from build123d import *

# Parameters (mm, degrees)
F0_W     = 25.4
F0_H     = 25.4
F1_DEPTH = 101.6
F3_DEPTH = 4.7625
F5_COUNT = 4
F5_ANGLE = 270


with BuildPart() as f1:
    # F0 (on Top) → F1 (new body)
    with BuildSketch(Plane.XY):
        Rectangle(F0_W, F0_H)
    extrude(amount=-F1_DEPTH)

    # F2 (on Right) → F3 (join, symmetric)
    with BuildSketch(Plane.YZ):
        Polygon((-88.9, -101.6), (-12.7, -101.6), (-12.7, -63.5), (-88.9, -95.25), align=None)
        Polygon((-15.3570100665, -67.4855150998), (-15.3570100665, -98.9429899335), (-86.2429899335, -98.9429899335), (-86.2429899335, -97.0213400443), align=None, mode=Mode.SUBTRACT)
    extrude(amount=F3_DEPTH, both=True)

    # F5: F1 ×4 about axis
    f5_axis = Axis((0, 0, -52.7451187372), (0, 0, -1))


with BuildPart() as f1_1:
    add(f1.part)
    for i in range(1, F5_COUNT):
        add(f1.part.rotate(f5_axis, i * F5_ANGLE / (F5_COUNT - 1)))


solid = f1_1.part
For this review, take the finished solid that the model builds, in its own axes (mm). A direction names the side the tool comes from. Round coordinates to 2 decimals unless told otherwise and drop trailing zeros. Loops run counter-clockwise (first coordinate to the right, second up) from the corner with the lowest first, then second, coordinate; pieces in that order, holes last. Notation, with made-up numbers: (17, 7.25) - (53, 7.25) arc R31 ccw to (53, 38.25) - close; hole circle Ø4 at (50.5, 20.25). An arc over 180 degrees is marked (long way). Use one line per item in the form item = value.
1) Tool access review of faces 5 (the face through (-12.7, 0, -50)), 6 (the face through (0, 12.7, -50)), 7 (the face through (15.357, 0, -83)), 8 (the face through (4.762, 48.2, -81)), 9 (the face through (-48.2, -4.763, -81)): name each direction out of +Z, -Z, +X, -X, +Y, -Y from which nothing blocks a thin tool from reaching the whole face with its end or side.
Solutions:
face_5 = +Z, -X
face_6 = +Z, +Y
face_7 = +Y, -Y
face_8 = +Z, -Z, +X, +Y
face_9 = +Z, -Z, -X, -Y
2) Wall thickness on probe 1 along Y at (x, z) = (8, -79.5); probe 2 along Z at (x, y) = (3.5, -52) (3 decimals): over which ranges is each line inside the solid? List them lowest first.
Solutions:
probe_1 = -12.7 to 12.7
probe_2 = -101.6 to -98.943, -82.753 to -79.875
3) Clearance check with flat-ended pins moving along their axes: P1, Ø3, axis at y = 1, z = -78, coming from the +X side; P2, Ø20.5, axis at y = -0.5, z = -30.5, coming from the -X side; P3, Ø19, axis at y = 57, z = -74.5, coming from the -X side; P4, Ø10.5, axis at y = 1, z = -90.5, coming from the -X side. State where each tip first meets the part, or that it passes through.
Solutions:
P1 = 51.1
P2 = -12.7
P3 = -4.76
P4 = -88.9
4) We need section B-B on y = -69.5. Write out the cut boundary in (x, z), then the cut area to 3 significant figures.
Solutions:
outline = (-4.76, -101.6) - (4.76, -101.6) - (4.76, -98.94) - (-4.76, -98.94) - close; (-4.76, -90.05) - (4.76, -90.05) - (4.76, -87.17) - (-4.76, -87.17) - close
area = 52.7 mm2
5) Mouldability with a two-part tool opening along Z and no side actions: class faces 1 (the face through (0, 0, 0)), 2 (the face through (12.7, 0, -50)), 3 (the face through (51.3, 0.07, -82.46)), 4 (the face through (0, -15.357, -83)) as pulls with the +Z half, pulls with the -Z half, needs draft (parallel to the pull), parting line crosses it, or undercut.
Solutions:
face_1 = pulls with the +Z half
face_2 = needs draft
face_3 = undercut
face_4 = undercut
6) We need section A-A on x = -32. Write out the cut boundary in (y, z), then the cut area to 3 significant figures.
Solutions:
outline = (-4.76, -101.6) - (4.76, -101.6) - (4.76, -98.94) - (-4.76, -98.94) - close; (-4.76, -74.42) - (4.76, -74.42) - (4.76, -71.54) - (-4.76, -71.54) - close
area = 52.7 mm2
7) We need section C-C on z = -33.5. Write out the cut boundary in (x, y).
Solutions:
outline = (-12.7, -12.7) - (12.7, -12.7) - (12.7, 12.7) - (-12.7, 12.7) - close
8) We need section D-D on z = -71.5. State how many separate pieces and enclosed holes the cut face has, then the cut area to 3 significant figures.
Solutions:
separate_pieces = 5
enclosed_holes = 0
area = 1,010 mm2
